Can you work these out from the drawing? Everything is in mm from the part's minimum corner. A direction names the side the tool comes from. Give positions to 0.01 mm unless a question says otherwise; leave off trailing zeros. Order: outer loops, then holes, each group sorted by start corner. A loop starts at its lowest first (then second) coordinate and runs counter-clockwise, first axis right, second up. Notation, with made-up numbers: M -23.5,-37.75 L 14.5,-37.75 A33 cw 14.5,-6.75 Z; hole C -20,77.25 d3. An arc over 180 degrees is marked long. Use a Markdown table: item, result. Add a question column.
Item 1: Suppose I cut it at B-B on y = 88. Write out the boundary of the cut face in (x, z).
Item 2: I'm going to push flat-ended pins straight in: pin 1 Ø4 at (x, z) = (225, 320) entering from +Y; pin 2 Ø1.9 at (x, y) = (135, 77.5) entering from -Z; pin 3 Ø5 at (y, z) = (97, 472) entering from +X. Where does each tip first touch, or does it pass through?
Item 3: If we mould it in two halves opening along X, with no side actions, what happens to the marked faces 1, 2 and 3? For each: released by +X, released by -X, zero draft, split by the parting line, or undercut.
Item 4: Suppose I cut it at A-A on x = 177.5. Write out the boundary of the cut face in (y, z).
Item 5: Suppose I cut it at C-C on x = 349.25. Write out the boundary of the cut face in (y, z).
Item 6: If I drill on L1, parallel to Y at x = 318, z = 277; L2, parallel to X at y = 166.5, z = 345; L3, parallel to Z at x = 397.5, y = 115.5, over which ranges is the centre line in solid material (lowest first)? Write a range as from..to.
Item 7: Suppose I cut it at D-D on z = 257. Write out the boundary of the cut face in (x, y), plus the area to 3 significant figures.
Item 8: For the marked faces 4, 5 and 6, which set-ups out of +Z, -Z, +X, -X, +Y, -Y let a thin tool reach every point of the face, with its end or its side?
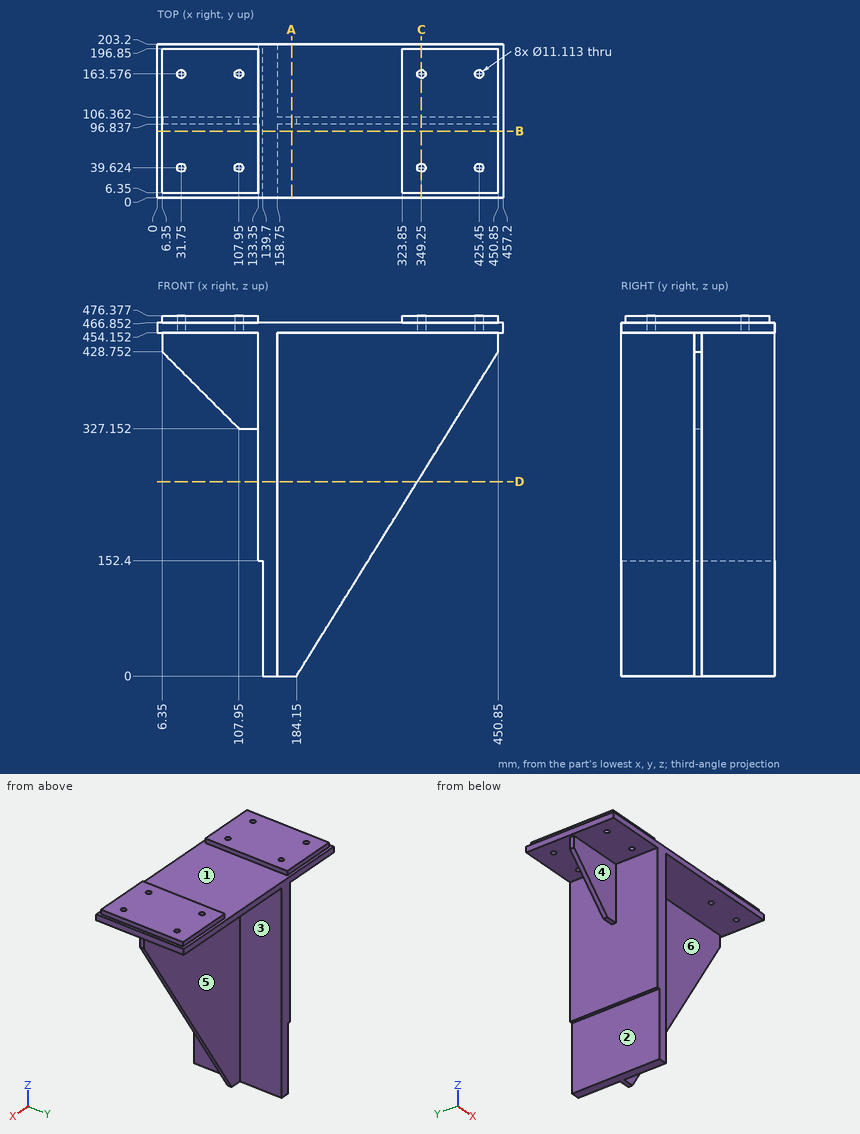
Findings below:
| question | item | result |
|---|---|---|
| 1 | outline | M 0,454.15 L 133.35,454.15 L 133.35,152.4 L 139.7,152.4 L 139.7,0 L 158.75,0 L 158.75,454.15 L 457.2,454.15 L 457.2,466.85 L 450.85,466.85 L 450.85,476.38 L 323.85,476.38 L 323.85,466.85 L 133.35,466.85 L 133.35,476.38 L 6.35,476.38 L 6.35,466.85 L 0,466.85 Z |
| 2 | pin 1 | stops at y = 106.36 |
| 2 | pin 2 | stops at z = 152.4 |
| 2 | pin 3 | stops at x = 450.85 |
| 3 | face 1 | undercut |
| 3 | face 2 | released by -X |
| 3 | face 3 | released by +X |
| 4 | outline | M 0,454.15 L 96.84,454.15 L 96.84,0 L 106.36,0 L 106.36,454.15 L 203.2,454.15 L 203.2,466.85 L 0,466.85 Z |
| 5 | outline | M 0,454.15 L 34.07,454.15 L 34.07,476.38 L 6.35,476.38 L 6.35,466.85 L 0,466.85 Z; M 45.18,454.15 L 96.84,454.15 L 96.84,265.42 L 106.36,265.42 L 106.36,454.15 L 158.02,454.15 L 158.02,476.38 L 45.18,476.38 Z; M 169.13,454.15 L 203.2,454.15 L 203.2,466.85 L 196.85,466.85 L 196.85,476.38 L 169.13,476.38 Z |
| 6 | L1 | y = 96.84..106.36 |
| 6 | L2 | x = 133.35..158.75 |
| 6 | L3 | z = 454.15..476.38 |
| 7 | outline | M 133.35,0 L 158.75,0 L 158.75,96.84 L 344.01,96.84 L 344.01,106.36 L 158.75,106.36 L 158.75,203.2 L 133.35,203.2 Z |
| 7 | area | 6,930 mm^2 |
| 8 | face 4 | -Z, -X, -Y |
| 8 | face 5 | -Z, +X, +Y |
| 8 | face 6 | -Z, +X, -Y |
